For this review, use the dimensioned drawing (mm, ordinates from the lowest corner) and the shaded views. A direction names the side the tool comes from. Coordinates: 2 decimals unless noted, no trailing zeros. Loops run counter-clockwise (first coordinate to the right, second up) from the corner with the lowest first, then second, coordinate; pieces in that order, holes last. Notation, with made-up numbers: (70.25, 15.25) -> (98.25, 15.25) arc R27 cw to (98.25, 40.25) -> close; hole circle Ø10 at (45.5, 9). An arc over 180 degrees is marked (long way). One line per question, with ' | ' between items. Start each with the question number.
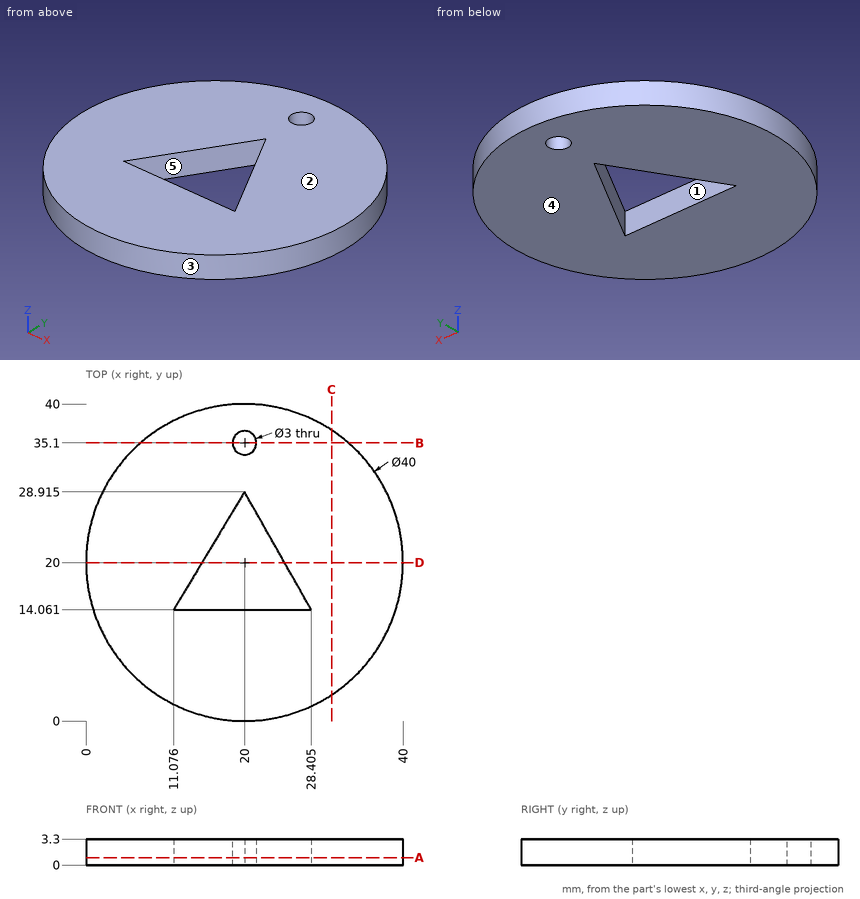
1) Consider section A-A, the plane z = 0.95. Write out the cut boundary in (x, y) (1 decimal).
2) Mouldability with a two-part tool opening along Y and no side actions: class the marked faces 3, 4 and 5 as +Y half, -Y half, draft (parallel to the pull), parting line (faces both ways), or undercut.
3) Consider section C-C, the plane x = 31. Write out the cut boundary in (y, z), plus the area to 3 significant figures.
4) Consider section D-D, the plane y = 20. Write out the cut boundary in (x, z) (1 decimal).
5) Insertion check: pin 1 Ø1.6 at (x, z) = (22, 1.5) entering from +Y; pin 2 Ø1 at (y, z) = (27, 1.5) entering from -X (1 decimal); pin 3 Ø1.8 at (x, y) = (20, 35.1) entering from -Z. Each pin has a flat end and moves straight along its axis. Give the tip position at first contact, or say it passes through.
6) Machinability: for the marked faces 1 and 2, which of the approach directions +Z, -Z, +X, -X, +Y, -Y give a long, thin tool a straight path to every point of the face, cutting with its end or side? Answer none if there is none.
7) Consider section B-B, the plane y = 35.1. Write out the cut boundary in (x, z) (1 decimal).
8) Wall thickness on L1, parallel to Y at x = 22, z = 2.2; L2, parallel to X at y = 16, z = 2.8 (1 decimal); L3, parallel to Y at x = 14, z = 0.5 (1 decimal): over which ranges is each line inside the solid? List them lowest first.
Filled sheet:
1) outline: circle Ø40 at (20, 20); hole (11.1, 14.1) -> (28.4, 14.1) -> (20, 28.9) -> close; hole circle Ø3 at (20, 35.1)
2) face 3: parting line | face 4: draft | face 5: undercut
3) outline: (3.3, 0) -> (36.7, 0) -> (36.7, 3.3) -> (3.3, 3.3) -> close | area: 110 mm^2
4) outline: (0, 0) -> (14.6, 0) -> (14.6, 3.3) -> (0, 3.3) -> close; (25, 0) -> (40, 0) -> (40, 3.3) -> (25, 3.3) -> close
5) pin 1: y = 39.96 | pin 2: x = 1.1 | pin 3: through
6) face 1: +Z, -Z | face 2: +Z, +X, -X, +Y, -Y
7) outline: (6.9, 0) -> (18.5, 0) -> (18.5, 3.3) -> (6.9, 3.3) -> close; (21.5, 0) -> (33.1, 0) -> (33.1, 3.3) -> (21.5, 3.3) -> close
8) L1: 0.1 to 14.06, 25.38 to 39.9 | L2: 0.4 to 12.2, 27.3 to 39.6 | L3: 0.9 to 14.1, 18.9 to 39.1
